Read the model definition and answer for the solid it produces. Units are mm, in the model's axes. A direction names the side the tool comes from. Give positions to 0.01 mm unless a question says otherwise; leave off trailing zeros. Loops run counter-clockwise (first coordinate to the right, second up) from the corner with the lowest first, then second, coordinate; pieces in that order, holes last. Notation, with made-up numbers: (19.5, 83.25) - (69.5, 83.25) arc R9 ccw to (69.5, 100.25) - close; hole circle Ø6 at (43.5, -2). An arc over 180 degrees is marked (long way). Write each question's results on one line, items separated by ' | '. Start each with the question number.
Q1. Given pin 1 (0.7 mm diameter, centred on y = 11, z = -13, fed in from +X); pin 2 (5 mm diameter, centred on x = 51, z = -10.5, fed in from +Y); pin 3 (5 mm diameter, centred on x = 49, y = 6, fed in from +Z); pin 4 (1.2 mm diameter, centred on x = 34, y = -12, fed in from +Z), each flat-ended and moving along its own axis, determine where each tip first touches the part or whether it passes through.
Q2. Determine the mould class of faces 4 (the flat face through (64.73, 11, -13)), 5 (the flat face through (58, -7.653, -17)), 6 (the flat face through (49, -10.153, -13)) for opening direction Y: +Y half, -Y half, draft (parallel to the pull), parting line (faces both ways), or undercut.
Q3. The part is cut by section A-A, the plane y = 4.75. Write down the section's boundary in (x, z), plus the area to 3 significant figures.
Q4. Find the intervals of material crossed by line 1 (Y direction, x = 55, z = -11.25); line 2 (Z direction, x = 65.5, y = 11.75); line 3 (Z direction, x = 72.5, y = -4), in increasing order. Write a range as from..to.
Q5. For faces 1 (the flat face through (59.906, 11, -13)), 2 (the flat face through (41, 10.153, -13)), 3 (the flat face through (41, 12.583, -13)), determine the directions among +Z, -Z, +X, -X, +Y, -Y from which every point of the face is accessible in a straight line to the end or side of a thin tool.
Q6. The part is cut by section C-C, the plane z = -17.75. Write down the section's boundary in (x, y).
Q7. The part is cut by section B-B, the plane z = -15.5. Write down the section's boundary in (x, y), plus the area to 3 significant figures.
```python
from build123d import *

# Parameters (mm, degrees)
SKETCH024_W                = 51.5
SKETCH024_H                = 14
SKETCH024_R                = 1.522099
SKETCH024_R_2              = 1.478889
PAD010_DEPTH               = 2
SKETCH025_W                = 18
SKETCH025_H                = 7.653357
PAD011_DEPTH               = 3
SKETCH026_W                = 2.323802
SKETCH026_H                = 2.429561
PAD012_DEPTH               = 5
SKETCH027_R                = 0.25
PAD013_DEPTH               = 10
SKETCH026_MIRRORED008_2_W  = 2.323802
SKETCH026_MIRRORED008_2_H  = 2.429561
PAD012_MIRRORED008_2_DEPTH = 5
SKETCH027_MIRRORED008_2_R  = 0.25
PAD013_MIRRORED008_2_DEPTH = 10
LINEARPATTERN_COUNT        = 15
LINEARPATTERN_PITCH        = 2.5


with BuildPart() as part:
    # Sketch024 → Pad010 (new body)
    with BuildSketch(Plane.XY):
        with Locations((-0.6866653219, 7)):
            Rectangle(SKETCH024_W, SKETCH024_H)
        with Locations((22.950167, 10.969199)):
            Circle(SKETCH024_R, mode=Mode.SUBTRACT)
        with Locations((-23.887783, 10.969199)):
            Circle(SKETCH024_R_2, mode=Mode.SUBTRACT)
    pad010 = extrude(amount=PAD010_DEPTH)

    # Sketch025 → Pad011 (join)
    with BuildSketch(Plane.XY):
        with Locations((8.993963, 3.8266785)):
            Rectangle(SKETCH025_W, SKETCH025_H)
    pad011 = extrude(amount=-PAD011_DEPTH)

    # Sketch026 → Pad012 (join)
    with BuildSketch(Plane.XY):
        with Locations((19.568367, 11.3677635)):
            Rectangle(SKETCH026_W, SKETCH026_H)
    pad012 = extrude(amount=PAD012_DEPTH)

    # Sketch027 → Pad013 (join)
    with BuildSketch(Plane.XY):
        with Locations((19.568367, 11.3677635)):
            Circle(SKETCH027_R)
    pad013 = extrude(amount=PAD013_DEPTH)

    # Mirrored007: Pad010, Pad011 across Sketch024 H_Axis
    add(pad010.mirror(Plane.ZX))
    add(pad011.mirror(Plane.ZX))

    # Sketch026 Mirrored008 2 → Pad012 Mirrored008 2 (add)
    with BuildSketch(Plane(origin=(0, 0, 0), x_dir=(1, 0, 0), z_dir=(0, 0, -1))):
        with Locations((19.568367, 11.3677635)):
            Rectangle(SKETCH026_MIRRORED008_2_W, SKETCH026_MIRRORED008_2_H)
    pad012_mirrored008_2 = extrude(amount=-PAD012_MIRRORED008_2_DEPTH)

    # Sketch027 Mirrored008 2 → Pad013 Mirrored008 2 (add)
    with BuildSketch(Plane(origin=(0, 0, 0), x_dir=(1, 0, 0), z_dir=(0, 0, -1))):
        with Locations((19.568367, 11.3677635)):
            Circle(SKETCH027_MIRRORED008_2_R)
    pad013_mirrored008_2 = extrude(amount=-PAD013_MIRRORED008_2_DEPTH)

    # LinearPattern: Pad012, Pad013, Pad012 Mirrored008 2, Pad013 Mirrored008 2 ×15
    with Locations(*[(-i * LINEARPATTERN_PITCH, 0, 0) for i in range(1, LINEARPATTERN_COUNT)]):
        add(pad012)
        add(pad013)
        add(pad012_mirrored008_2)
        add(pad013_mirrored008_2)


with BuildPart() as part_1:
    # Body004 placement: moved
    add(part.part.moved(Location((49, 0, -16))))


solid = part_1.part
```
Check sheet entries:
1) pin 1: stops at x = 69.73 | pin 2: stops at y = 12.58 | pin 3: stops at z = -14 | pin 4: stops at z = -6
2) face 4: draft | face 5: -Y half | face 6: undercut
3) outline: (22.56, -16) - (48.99, -16) - (48.99, -19) - (66.99, -19) - (66.99, -16) - (74.06, -16) - (74.06, -14) - (22.56, -14) - close | area: 157 mm^2
4) line 1: y = -12.58..-10.15, 10.15..12.58 | line 2: z = -16..-11 | line 3: z = -16..-14
5) face 1: +Z, +Y, -Y | face 2: +Z, +X, -X | face 3: +Z, +X, -X, +Y
6) outline: (48.99, -7.65) - (66.99, -7.65) - (66.99, 7.65) - (48.99, 7.65) - close
7) outline: (22.56, -14) - (74.06, -14) - (74.06, 14) - (22.56, 14) - close; hole circle Ø2.96 at (25.11, -10.97); hole circle Ø2.96 at (25.11, 10.97); hole circle Ø3.04 at (71.95, -10.97); hole circle Ø3.04 at (71.95, 10.97) | area: 1,410 mm^2
